Verification items for this drawing (mm, ordinates from the low corner). Round coordinates to 2 decimals unless told otherwise and drop trailing zeros. Loops run counter-clockwise (first coordinate to the right, second up) from the corner with the lowest first, then second, coordinate; pieces in that order, holes last. Notation, with made-up numbers: (45, -34) - (93, -34) arc R12 cw to (93, -19) - close; hole circle Ø4 at (47.25, -21.5). An arc over 180 degrees is marked (long way). Put each result on its own line as item: value.
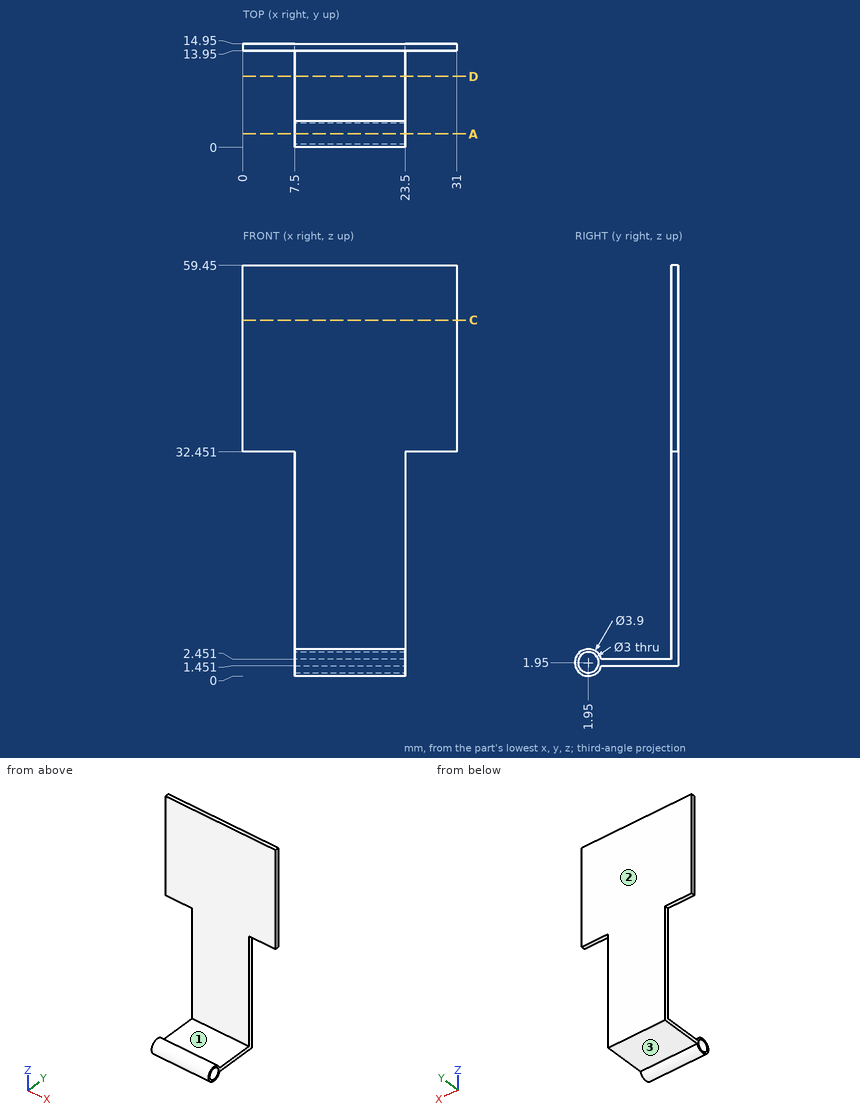
Item 1: Section check C-C on z = 51.5. Enter the section's corners in (x, y).
Filled sheet:
outline: (0, 13.95) - (31, 13.95) - (31, 14.95) - (0, 14.95) - close
Item 2: Section check A-A on y = 1.95. Enter the section's corners in (x, z).
Filled sheet:
outline: (7.5, 0) - (23.5, 0) - (23.5, 0.45) - (7.5, 0.45) - close; (7.5, 3.45) - (23.5, 3.45) - (23.5, 3.9) - (7.5, 3.9) - close
Item 3: Section check D-D on y = 10.25. Enter the section's corners in (x, z).
Filled sheet:
outline: (7.5, 1.45) - (23.5, 1.45) - (23.5, 2.45) - (7.5, 2.45) - close
Item 4: Thickness scan on line 1 (Y direction, x = 17.75, z = 1.95); line 2 (Y direction, x = 11.5, z = 26); line 3 (Z direction, x = 17, y = 7.25). Record the ranges inside material, lowest first. Write a range as from..to.
Filled sheet:
line 1: 0..0.45, 3.45..14.95
line 2: 13.95..14.95
line 3: 1.45..2.45
Item 5: Release check for a two-part mould opening along Y. For the marked faces 1, 2 and 3 record: +Y half, -Y half, draft (parallel to the pull), parting line (faces both ways), or undercut.
Filled sheet:
face 1: undercut
face 2: +Y half
face 3: draft
Item 6: Go/stop test with flat-tipped pins: pin 1 (7.5 mm diameter, centred on y = 10, z = 16.5, fed in from +X); pin 2 (15.5 mm diameter, centred on x = 23, z = 44, fed in from -Y); pin 3 (8 mm diameter, centred on x = 14, y = 6.5, fed in from +Z); pin 4 (4 mm diameter, centred on y = 1.95, z = 1.95, fed in from -X). Record where each tip stops, or that it passes through.
Filled sheet:
pin 1: through
pin 2: y = 13.95
pin 3: z = 3.82
pin 4: x = 7.5
